Part model, mm, in its own coordinate system. A direction names the side the tool comes from. Round coordinates to 2 decimals unless told otherwise and drop trailing zeros. Loops run counter-clockwise (first coordinate to the right, second up) from the corner with the lowest first, then second, coordinate; pieces in that order, holes last. Notation, with made-up numbers: (-37, 31) -> (-22, 31) arc R17 cw to (-22, 48) -> close; hole circle Ø4 at (30, -8.5). An arc over 180 degrees is marked (long way). Use a Markdown table: item, result. Add a question column.
Item 1: Which spindle directions (+Z, -Z, +X, -X, +Y, -Y) get a long thin tool onto all of the face, cutting with end or side? Do faces 5 (the face through (0, -2.5, 0)), 6 (the face through (-0.28, 6.73, 8.32)), 7 (the face through (0, -1, -1)). Say none if no direction does.
Item 2: Two-plate mould, pull along X, no slides. Class faces 1 (the face through (-1.5, 0, 0)), 2 (the face through (0, 8, 16)), 3 (the face through (-0.17, 2.54, -1.29)), 4 (the face through (0, 8, 14)): pulls with the +X half, pulls with the -X half, needs draft (parallel to the pull), parting line crosses it, or undercut.
Item 3: Cut at B-B, the plane z = 5.5. List the corners of the cut face in (x, y).
Item 4: Flat gauge pins, fed straight in: pin 1 (1.3 mm diameter, centred on x = -0.5, z = 0.5, fed in from +Y); pin 2 (1.3 mm diameter, centred on x = -1, y = 7.5, fed in from +Z); pin 3 (1 mm diameter, centred on y = 5.5, z = 9, fed in from +X); pin 4 (0.5 mm diameter, centred on x = 0, y = 9.5, fed in from +Z). Where does each tip first touch, or does it go through?
Item 5: Probe line 1 (X direction, y = 8, z = 14.45); line 2 (Y direction, x = 0, z = 14.1); line 3 (Y direction, x = -1.55, z = 0.5). List the from-to ranges inside material, lowest first. Write a range as [from, to].
Item 6: Cut at A-A, the plane y = -0.75. List the corners of the cut face in (x, z).
```python
from build123d import *

# Parameters (mm, degrees)
F1_R             = 1.3
F3_W             = 4.4
F3_H             = 4.4
F3_R             = 1.3
F4_DEPTH         = 0.5
F5_R             = 1
F6_DEPTH         = 2
F7_R             = 0.2
F8_R             = 1.6
F8_R_2           = 1.3
F9_DEPTH         = 0.5
F9_DEPTH_BACK    = 0.5
F11_DEPTH        = 1.5
F11_COPIES_COUNT = 3


# Not quite as in the source:
# - a pattern or mirror of a feature is missing from the dataset's text; its kind, count and spacing are read off the source's solid


with BuildPart() as f2:
    # F2: sweep along a path in F0
    with BuildLine(Plane.YZ) as f2_path:
        Line((0, 0), (5, 0))
        ThreePointArc((5, 0), (7.1213203436, 0.8786796564), (8, 3))
        Line((8, 3), (8, 14))
    # F1 (on Front) → F2 (sweep)
    with BuildSketch(Plane.XZ):
        Circle(F1_R)
    sweep(path=f2_path.line)

    # F3 (on face) → F4 (join)
    with BuildSketch(Plane.XZ):
        Rectangle(F3_W, F3_H)
        Circle(F3_R, mode=Mode.SUBTRACT)
        Circle(F3_R)
    extrude(amount=F4_DEPTH)

    # F5 (on face) → F6 (join)
    with BuildSketch(Plane.XZ.offset(0.5)):
        Circle(F5_R)
    extrude(amount=F6_DEPTH)

    # F7
    f7_edges = [f2.edges().sort_by_distance(p)[0] for p in [
        (-1, -2.5, 0),
    ]]
    fillet(f7_edges, radius=F7_R)

    # F8 (on face) → F9 (join, two sides)
    with BuildSketch(Plane.XY.offset(14)) as f9_sk:
        with Locations((0, 8)):
            Circle(F8_R)
        with Locations((0, 8)):
            Circle(F8_R_2, mode=Mode.SUBTRACT)
    extrude(amount=-F9_DEPTH)
    extrude(f9_sk.sketch, amount=F9_DEPTH_BACK)

    # F10 (on face) → F11 (join)
    with BuildSketch(Plane.XY.offset(14.5)):
        with BuildLine():
            Line((-0.4, 6.7630683123), (-0.4, 6.4508066615))
            ThreePointArc((-0.4, 6.4508066615), (0, 6.4), (0.4, 6.4508066615))
            Line((0.4, 6.4508066615), (0.4, 6.7630683123))
            ThreePointArc((0.4, 6.7630683123), (0, 6.7), (-0.4, 6.7630683123))
        make_face()
    f11 = extrude(amount=F11_DEPTH)

    # F11_copies: F11 ×3 about axis
    f11_copies_axis = Axis((0, 8, 0), (0, 0, 1))
    for i in range(1, F11_COPIES_COUNT):
        add(f11.rotate(f11_copies_axis, i * 360 / F11_COPIES_COUNT))

    # F13 (on Right) → F14 (revolve)
    with BuildSketch(Plane.YZ):
        Polygon((6, 16), (6.4508066615, 16), (6.7630683123, 16), (8, 16), (8, 18), align=None)
    revolve(axis=Axis((0, 8, 17.9220158607), (0, 0, 1)))


solid = f2.part
```
A:
| question | item | result |
|---|---|---|
| 1 | face 5 | +Z, -Z, +X, -X, -Y |
| 1 | face 6 | none |
| 1 | face 7 | -Y |
| 2 | face 1 | needs draft |
| 2 | face 2 | undercut |
| 2 | face 3 | parting line crosses it |
| 2 | face 4 | undercut |
| 3 | outline | circle Ø2.6 at (0, 8) |
| 4 | pin 1 | stops at y = 8.83 |
| 4 | pin 2 | stops at z = 17.53 |
| 4 | pin 3 | passes through |
| 4 | pin 4 | stops at z = 16.75 |
| 5 | line 1 | x = [-1.6, -1.3], [1.3, 1.6] |
| 5 | line 2 | y = [6.4, 6.7], [9.3, 9.6] |
| 5 | line 3 | y = [-0.5, 0] |
| 6 | outline | circle Ø2 at (0, 0) |
